```python
from build123d import *

# Parameters (mm, degrees)
SKETCH9_W                           = 12
SKETCH9_H                           = 40.19
EXTRUDE3_DEPTH                      = 7
F_3_32_0_09375_DIAMETER_HOLE1_D     = 2.38125
F_3_32_0_09375_DIAMETER_HOLE1_DEPTH = 10
F_3_32_0_09375_DIAMETER_HOLE1_TIP   = 0.715399675
F_6_0_6_DIAMETER_HOLE1_D            = 6
F_6_0_6_DIAMETER_HOLE1_DEPTH        = 10
F_6_0_6_DIAMETER_HOLE1_TIP          = 1.802581857
F_6_32_TAPPED_HOLE2_D               = 2.7051
F_6_32_TAPPED_HOLE2_DEPTH           = 7.9624
F_6_32_TAPPED_HOLE2_TIP             = 0.81269403
F_6_32_TAPPED_HOLE1_D               = 2.7051
F_6_32_TAPPED_HOLE1_DEPTH           = 9.96
F_6_32_TAPPED_HOLE1_TIP             = 0.81269403


with BuildPart() as part:
    # Sketch9 → Extrude3 (new body)
    with BuildSketch(Plane(origin=(0, 0, 0), x_dir=(1, 0, 0), z_dir=(0, 1, 0))):
        Rectangle(SKETCH9_W, SKETCH9_H)
    extrude(amount=EXTRUDE3_DEPTH)

    # 3/32 (0.09375) Diameter Hole1
    with Locations(Plane(origin=(-0.08113915, 7, -13.266251032), x_dir=(0, 0, 1), z_dir=(0, 1, 0))):
        with Locations((0, 0)):
            Hole(F_3_32_0_09375_DIAMETER_HOLE1_D / 2, depth=F_3_32_0_09375_DIAMETER_HOLE1_DEPTH)
            with Locations((0, 0, -(F_3_32_0_09375_DIAMETER_HOLE1_DEPTH + F_3_32_0_09375_DIAMETER_HOLE1_TIP / 2))):  # 118° drill point
                Cone(0, F_3_32_0_09375_DIAMETER_HOLE1_D / 2, F_3_32_0_09375_DIAMETER_HOLE1_TIP, mode=Mode.SUBTRACT)

    # Ø6.0 (6) Diameter Hole1
    with Locations(Plane(origin=(0, 7, 13.266499161), x_dir=(0, 0, 1), z_dir=(0, 1, 0))):
        with Locations((0, 0)):
            Hole(F_6_0_6_DIAMETER_HOLE1_D / 2, depth=F_6_0_6_DIAMETER_HOLE1_DEPTH)
            with Locations((0, 0, -(F_6_0_6_DIAMETER_HOLE1_DEPTH + F_6_0_6_DIAMETER_HOLE1_TIP / 2))):  # 118° drill point
                Cone(0, F_6_0_6_DIAMETER_HOLE1_D / 2, F_6_0_6_DIAMETER_HOLE1_TIP, mode=Mode.SUBTRACT)

    # #6-32 Tapped Hole2
    with Locations(Plane(origin=(0, 3.5, 20.095), x_dir=(1, 0, 0), z_dir=(0, 0, 1))):
        with Locations((0, 0)):
            Hole(F_6_32_TAPPED_HOLE2_D / 2, depth=F_6_32_TAPPED_HOLE2_DEPTH)
            with Locations((0, 0, -(F_6_32_TAPPED_HOLE2_DEPTH + F_6_32_TAPPED_HOLE2_TIP / 2))):  # 118° drill point
                Cone(0, F_6_32_TAPPED_HOLE2_D / 2, F_6_32_TAPPED_HOLE2_TIP, mode=Mode.SUBTRACT)

    # #6-32 Tapped Hole1
    with Locations(Plane(origin=(0, 3.5, -20.095), x_dir=(-1, 0, 0), z_dir=(0, 0, -1))):
        with Locations((0, 0)):
            Hole(F_6_32_TAPPED_HOLE1_D / 2, depth=F_6_32_TAPPED_HOLE1_DEPTH)
            with Locations((0, 0, -(F_6_32_TAPPED_HOLE1_DEPTH + F_6_32_TAPPED_HOLE1_TIP / 2))):  # 118° drill point
                Cone(0, F_6_32_TAPPED_HOLE1_D / 2, F_6_32_TAPPED_HOLE1_TIP, mode=Mode.SUBTRACT)


solid = part.part
```
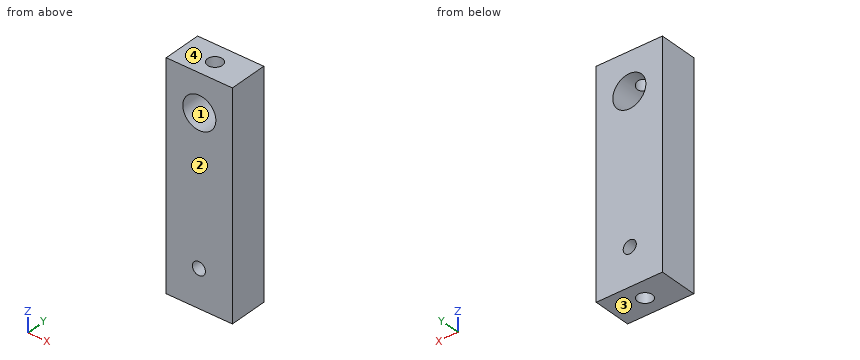
Build history of the part. All positions in model axes, mm. Face numbers are marked on the shaded views. Give positions to 0.01 mm unless a question says otherwise; leave off trailing zeros. Loops run counter-clockwise (first coordinate to the right, second up) from the corner with the lowest first, then second, coordinate; pieces in that order, holes last. Notation, with made-up numbers: (-10.75, 28.5) -> (40.25, 28.5) arc R37 ccw to (40.25, 65.5) -> close; hole circle Ø5 at (52.25, 32.25). An arc over 180 degrees is marked (long way). One line per question, with ' | ' between items. Start each with the question number.
1) Pin check, flat tips, straight feed: pin 1 (3.5 mm diameter, centred on x = 0, z = 13.27, fed in from -Y); pin 2 (2.5 mm diameter, centred on x = 0, y = 3.5, fed in from -Z); pin 3 (3.5 mm diameter, centred on x = 0, y = 3.5, fed in from -Z) (3 decimals). Stop position of each tip, or through.
2) Cut at A-A (z = -10.5). Give the cut face in (x, y).
3) Two-plate mould, pull along Z, no slides. Class the marked faces 1, 2, 3 and 4: released by +Z, released by -Z, zero draft, split by the parting line, or undercut.
4) Probe L1, parallel to Z at x = 0, y = 5 (1 decimal); L2, parallel to Z at x = 0.5, y = 2 (3 decimals); L3, parallel to Y at x = 0, z = 17.4. List the from-to ranges inside material, lowest first.
5) Cut at B-B (y = 5.5). Give the cut face in (x, z) (1 decimal), plus the area to 3 significant figures.
Return value:
1) pin 1: through | pin 2: z = -10.07 | pin 3: z = -20.095
2) outline: (-6, 0) -> (6, 0) -> (6, 7) -> (-6, 7) -> close; hole circle Ø2.71 at (0, 3.5)
3) face 1: undercut | face 2: zero draft | face 3: released by -Z | face 4: released by +Z
4) L1: -20.1 to -14.5, -12.1 to 10.3, 16.3 to 20.1 | L2: -20.095 to -14.305, -12.227 to 10.308, 16.225 to 20.095 | L3: 0 to 2.15, 4.85 to 7
5) outline: (-6, -20.1) -> (6, -20.1) -> (6, 20.1) -> (-6, 20.1) -> close; hole circle Ø6 at (0, 13.3); hole circle Ø2.4 at (-0.1, -13.3) | area: 450 mm^2
